Here's the drawing with two shaded views (mm, measured from the low corner). I have some questions. Coordinates: 2 decimals unless noted, no trailing zeros. Write each loop counter-clockwise with the first axis right and the second up, starting at its lowest first coordinate (ties: lowest second). Pieces come first, ordered by that corner, then holes.
Item 1: If we section it at B-B (y = 36.6): Please give me the cut outline in (x, z), then the cut area to 3 significant figures.
Item 2: I'm going to push a flat-ended pin straight in: pin 1 Ø6 at (y, z) = (13, 5) entering from +X. Where does the tip first touch, or does it pass through?
Item 3: If I drill on line 1 (Y direction, x = 1.8, z = 9); line 2 (Z direction, x = 2.45, y = 16.5); line 3 (Y direction, x = 0.3, z = 7.25), over which ranges is the centre line in solid material (lowest first)?
Item 4: If we section it at D-D (y = 56.7): Please give me the cut outline in (x, z), then the cut area to 3 significant figures.
Item 5: If we section it at C-C (x = 0.5): Please give me the cut outline in (y, z).
Item 6: If we section it at A-A (z = 9): Please give me the cut outline in (x, y), then the cut area to 3 significant figures.
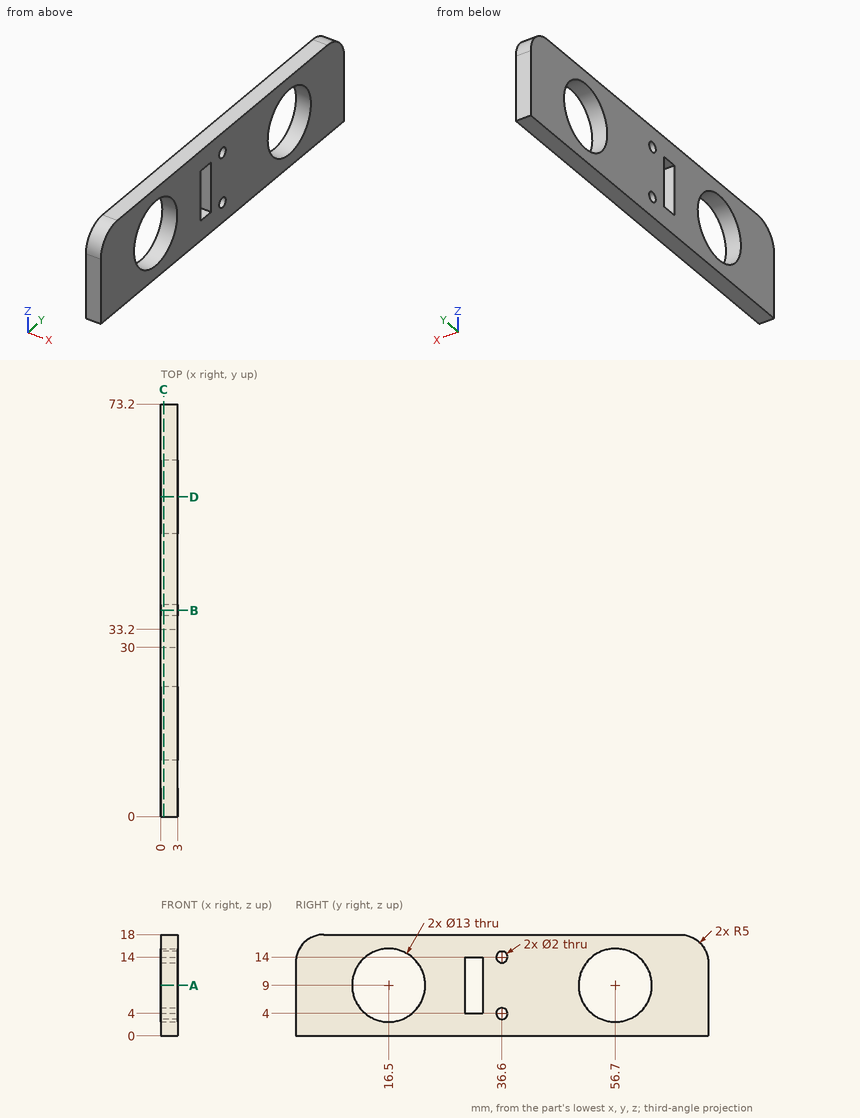
Answer list:
1. outline: (0, 0) - (3, 0) - (3, 3) - (0, 3) - close; (0, 5) - (3, 5) - (3, 13) - (0, 13) - close; (0, 15) - (3, 15) - (3, 18) - (0, 18) - close
1. area: 42.0 mm2
2. pin 1: stops at x = 3
3. line 1: y = 0 to 10, 23 to 30, 33.2 to 50.2, 63.2 to 73.2
3. line 2: z = 0 to 2.5, 15.5 to 18
3. line 3: y = 0 to 10.24, 22.76 to 30, 33.2 to 50.44, 62.96 to 73.2
4. outline: (0, 0) - (3, 0) - (3, 2.5) - (0, 2.5) - close; (0, 15.5) - (3, 15.5) - (3, 18) - (0, 18) - close
4. area: 15.0 mm2
5. outline: (0, 0) - (73.2, 0) - (73.2, 13) arc R5 ccw to (68.2, 18) - (5, 18) arc R5 ccw to (0, 13) - close; hole circle Ø13 at (16.5, 9); hole (30, 4) - (33.2, 4) - (33.2, 14) - (30, 14) - close; hole circle Ø2 at (36.6, 4); hole circle Ø2 at (36.6, 14); hole circle Ø13 at (56.7, 9)
6. outline: (0, 0) - (3, 0) - (3, 10) - (0, 10) - close; (0, 23) - (3, 23) - (3, 30) - (0, 30) - close; (0, 33.2) - (3, 33.2) - (3, 50.2) - (0, 50.2) - close; (0, 63.2) - (3, 63.2) - (3, 73.2) - (0, 73.2) - close
6. area: 132 mm2
